For this review, take the finished solid that the model builds, in its own axes (mm). A direction names the side the tool comes from. Coordinates: 2 decimals unless noted, no trailing zeros. Loops run counter-clockwise (first coordinate to the right, second up) from the corner with the lowest first, then second, coordinate; pieces in that order, holes last. Notation, with made-up numbers: (27, 69.25) -> (60, 69.25) arc R24 ccw to (60, 85.25) -> close; hole circle Ø7 at (55.5, 80.5). An arc over 180 degrees is marked (long way). One line per item, written item: value.
from build123d import *

# Parameters (mm, degrees)
SKETCH1_W           = 10
SKETCH1_H           = 10
SKETCH1_W_2         = 44
SKETCH1_H_2         = 44
BOSS_EXTRUDE1_DEPTH = 2
BOSS_EXTRUDE2_DEPTH = 30
CUT_EXTRUDE1_DEPTH  = 12
CUT_EXTRUDE2_DEPTH  = 12
FILLET1_R           = 5


with BuildPart() as part:
    # Sketch1 → Boss-Extrude1 (new body)
    with BuildSketch(Plane.XY):
        Rectangle(SKETCH1_W, SKETCH1_H)
        with Locations((-27, 0)):
            Rectangle(SKETCH1_W_2, SKETCH1_H)
        with Locations((0, 27)):
            Rectangle(SKETCH1_W, SKETCH1_H_2)
        with Locations((27, 0)):
            Rectangle(SKETCH1_W_2, SKETCH1_H)
        with Locations((0, -27)):
            Rectangle(SKETCH1_W, SKETCH1_H_2)
    extrude(amount=BOSS_EXTRUDE1_DEPTH)

    # Sketch3 → Boss-Extrude2 (add)
    with BuildSketch(Plane(origin=(0, 0, 0), x_dir=(-1, 0, 0), z_dir=(0, 0, -1))):
        with BuildLine():
            Line((-48.744230428, 5), (-40.794730052, 5))
            ThreePointArc((-40.794730052, 5), (-41.1, 0), (-40.794730052, -5))
            Line((-40.794730052, -5), (-48.744230428, -5))
            ThreePointArc((-48.744230428, -5), (-49, 0), (-48.744230428, 5))
        make_face()
        with BuildLine():
            Line((5, 48.744230428), (5, 40.794730052))
            ThreePointArc((5, 40.794730052), (0, 41.1), (-5, 40.794730052))
            Line((-5, 40.794730052), (-5, 48.744230428))
            ThreePointArc((-5, 48.744230428), (0, 49), (5, 48.744230428))
        make_face()
        with BuildLine():
            Line((48.744230428, -5), (40.794730052, -5))
            ThreePointArc((40.794730052, -5), (41.1, 0), (40.794730052, 5))
            Line((40.794730052, 5), (48.744230428, 5))
            ThreePointArc((48.744230428, 5), (49, 0), (48.744230428, -5))
        make_face()
        with BuildLine():
            Line((-5, -48.744230428), (-5, -40.794730052))
            ThreePointArc((-5, -40.794730052), (0, -41.1), (5, -40.794730052))
            Line((5, -40.794730052), (5, -48.744230428))
            ThreePointArc((5, -48.744230428), (0, -49), (-5, -48.744230428))
        make_face()
    extrude(amount=BOSS_EXTRUDE2_DEPTH)

    # Sketch4 → Cut-Extrude1 (cut)
    with BuildSketch(Plane(origin=(0, 0, -30), x_dir=(-1, 0, 0), z_dir=(0, 0, -1))):
        with BuildLine():
            Line((-11.10557259, -44.484702511), (-11.461711595, -41.548034458))
            ThreePointArc((-11.461711595, -41.548034458), (-43.096967164, -0.511293704), (-12.444181806, 41.264419773))
            Line((-12.444181806, 41.264419773), (-14.129590932, 43.618541471))
            ThreePointArc((-14.129590932, 43.618541471), (-45.823015718, -1.572809738), (-11.10557259, -44.484702511))
        make_face()
        with BuildLine():
            Line((12.001150898, -44.251495762), (13.254659766, -41.011266677))
            ThreePointArc((13.254659766, -41.011266677), (43.094432914, 0.692713402), (11.929696672, 41.416087905))
            Line((11.929696672, 41.416087905), (17.322221173, 42.451892227))
            ThreePointArc((17.322221173, 42.451892227), (45.76389854, -2.80857445), (12.001150898, -44.251495762))
        make_face()
    extrude(amount=-CUT_EXTRUDE1_DEPTH, mode=Mode.SUBTRACT)

    # Sketch5 → Cut-Extrude2 (cut)
    with BuildSketch(Plane(origin=(0, 0, -30), x_dir=(-1, 0, 0), z_dir=(0, 0, -1))):
        with BuildLine():
            Line((-42.028433613, 16.76822197), (-39.816299645, 14.863118199))
            ThreePointArc((-39.816299645, 14.863118199), (-0.915555868, 42.490137179), (39.139115264, 16.564409328))
            Line((39.139115264, 16.564409328), (42.109177665, 16.564409328))
            ThreePointArc((42.109177665, 16.564409328), (0.109612038, 45.24986724), (-42.028433613, 16.76822197))
        make_face()
        with BuildLine():
            Line((-42.268216712, -16.154267422), (-39.699430061, -15.172516364))
            ThreePointArc((-39.699430061, -15.172516364), (-1.394243302, -42.477124263), (38.619024806, -17.743193711))
            Line((38.619024806, -17.743193711), (40.007756731, -21.141000481))
            ThreePointArc((40.007756731, -21.141000481), (-2.737571274, -45.167114182), (-42.268216712, -16.154267422))
        make_face()
    extrude(amount=-CUT_EXTRUDE2_DEPTH, mode=Mode.SUBTRACT)

    # Fillet1
    fillet1_edges = [part.edges().sort_by_distance(p)[0] for p in [
        (41.1, 0, 0),
        (0, 41.1, 0),
        (-41.1, 0, 0),
        (0, -41.1, 0),
    ]]
    fillet(fillet1_edges, radius=FILLET1_R)


solid = part.part
1. To check wall thickness, follow probe 1 along Y at (x, z) = (-1.5, -10.5); probe 2 along Z at (x, y) = (13, -2); probe 3 along Y at (x, z) = (-42.5, -2). State the ranges of each line that lie inside material, in increasing order. Write a range as from..to.
Return value:
probe 1: y = -48.98..-41.07, 41.07..48.98
probe 2: z = 0..2
probe 3: y = -5..5
2. Insertion check: pin 1 Ø3 at (y, z) = (38.5, -12.5) entering from -X; pin 2 Ø10 at (x, z) = (-6, -21) entering from +Y; pin 3 Ø0.9 at (x, y) = (2, 44) entering from -Z; pin 4 Ø1.5 at (x, z) = (4, -19) entering from -Y. Each pin has a flat end and moves straight along its axis. Give the tip position at first contact, or say it passes through.
Return value:
pin 1: passes through
pin 2: stops at y = 48.99
pin 3: stops at z = -18
pin 4: stops at y = -48.89
3. Take a section at C-C, the plane z = -3.5. Give the boundary of the cut face in (x, y).
Return value:
outline: (-48.74, -5) -> (-40.56, -5) arc R40.87 cw to (-40.56, 5) -> (-48.74, 5) arc R49 ccw to start; (-5, -48.74) arc R49 ccw to (5, -48.74) -> (5, -40.56) arc R40.87 cw to (-5, -40.56) -> close; (-5, 40.56) arc R40.87 cw to (5, 40.56) -> (5, 48.74) arc R49 ccw to (-5, 48.74) -> close; (40.56, -5) -> (48.74, -5) arc R49 ccw to (48.74, 5) -> (40.56, 5) arc R40.87 cw to start
4. Take a section at A-A, the plane z = -16. Give the boundary of the cut face in (x, y), and give its area (3 significant figures).
Return value:
outline: (-48.74, -5) -> (-40.79, -5) arc R41.1 cw to (-40.79, 5) -> (-48.74, 5) arc R49 ccw to start; (-5, -48.74) arc R49 ccw to (5, -48.74) -> (5, -40.79) arc R41.1 cw to (-5, -40.79) -> close; (-5, 40.79) arc R41.1 cw to (5, 40.79) -> (5, 48.74) arc R49 ccw to (-5, 48.74) -> close; (40.79, -5) -> (48.74, -5) arc R49 ccw to (48.74, 5) -> (40.79, 5) arc R41.1 cw to start
area: 317 mm2
5. Take a section at B-B, the plane y = -10. Give the boundary of the cut face in (x, z), and give its area (3 significant figures).
Return value:
outline: (-5, 0) -> (5, 0) -> (5, 2) -> (-5, 2) -> close
area: 20.0 mm2
6. The part is to be moulded in two halves that separate along Y. For faces 5 (the cylindrical face through (-45.85, 0.07, -24.08)), 6 (the flat face through (47, 0, -30)), 7 (the cylindrical face through (49, 0, -15)), 8 (the flat face through (42, -5, -8)), say which applies: pulls with the +Y half, pulls with the -Y half, needs draft (parallel to the pull), parting line crosses it, or undercut.
Return value:
face 5: undercut
face 6: needs draft
face 7: parting line crosses it
face 8: pulls with the -Y half
7. For faces 1 (the flat face through (5, 42, -8)), 2 (the cylindrical face through (-41.1, -0.1, -17.3)), 3 (the flat face through (-5, -42, -11)), 4 (the flat face through (-5, 42, -8)), list the 3-axis set-ups (+Z, -Z, +X, -X, +Y, -Y) from which the entire face can be reached by the end or side of a thin tool; tool diameter is ignored.
Return value:
face 1: +Z, -Z, +X, +Y
face 2: -Z
face 3: +Z, -Z, -X, -Y
face 4: +Z, -Z, -X, +Y
